from build123d import *

# Parameters (mm, degrees)
SKETCH2_W              = 127
SKETCH2_H              = 127
BOSS_EXTRUDE1_DEPTH    = 12.7
SKETCH3_W              = 38.1
SKETCH3_H              = 4.04158002
CUT_EXTRUDE2_DEPTH     = 128
F_10_0MM_DOWEL_HOLE1_D = 8.382
CUT_EXTRUDE4_DEPTH     = 13.7


with BuildPart() as part:
    # Sketch2 → Boss-Extrude1 (new body)
    with BuildSketch(Plane(origin=(0, 0, 0), x_dir=(1, 0, 0), z_dir=(0, 1, 0))):
        Rectangle(SKETCH2_W, SKETCH2_H)
    extrude(amount=BOSS_EXTRUDE1_DEPTH)

    # Sketch3 → Cut-Extrude2 (cut, through all)
    with BuildSketch(Plane.XY.offset(63.5)):
        with Locations((-44.45, 10.67920999)):
            Rectangle(SKETCH3_W, SKETCH3_H)
        with Locations((44.45, 10.67920999)):
            Rectangle(SKETCH3_W, SKETCH3_H)
    extrude(amount=-CUT_EXTRUDE2_DEPTH, mode=Mode.SUBTRACT)

    # Ø10.0mm Dowel Hole1 (through all)
    with Locations(Plane(origin=(0, 0, 0), x_dir=(-1, 0, 0), z_dir=(0, -1, 0))):
        with Locations((-44.45, 43.18), (-44.45, -4.572), (-44.45, -42.672), (44.45, 43.18), (44.45, -4.572), (44.45, -42.672)):
            Hole(F_10_0MM_DOWEL_HOLE1_D / 2)

    # Sketch10 → Cut-Extrude4 (cut, through all)
    with BuildSketch(Plane(origin=(0, 0, 0), x_dir=(-1, 0, 0), z_dir=(0, -1, 0))):
        with BuildLine():
            Line((7.62, -11.938), (7.62, -36.322))
            ThreePointArc((7.62, -36.322), (0, -43.942), (-7.62, -36.322))
            Line((-7.62, -36.322), (-7.62, -11.938))
            ThreePointArc((-7.62, -11.938), (0, -4.318), (7.62, -11.938))
        make_face()
    extrude(amount=-CUT_EXTRUDE4_DEPTH, mode=Mode.SUBTRACT)


solid = part.part
Can you work these out from the model? Positions are in its coordinate system, mm. A direction names the side the tool comes from. Round coordinates to 2 decimals unless told otherwise and drop trailing zeros. Write each loop counter-clockwise with the first axis right and the second up, starting at its lowest first coordinate (ties: lowest second). Pieces come first, ordered by that corner, then holes. Notation, with made-up numbers: (-10.5, -37.5) -> (41.5, -37.5) arc R30 ccw to (41.5, -7.5) -> close; hole circle Ø10 at (80.5, 63.25). An arc over 180 degrees is marked (long way). One line per question, with ' | ' between items. Start each with the question number.
1) If we mould it in two halves opening along Z, with no side actions, what happens to faces 1 (the flat face through (-1, 5, -63.5)), 2 (the flat face through (63.5, 4, 1)), 3 (the cylindrical face through (-47.78, 4.39, 45.22))? For each: released by +Z, released by -Z, zero draft, split by the parting line, or undercut.
2) Suppose I cut it at B-B on x = 0. Write out the boundary of the cut face in (y, z), then the cut area to 3 significant figures.
3) On a 3-axis mill with a long thin cutter (end or side, diameter ignored), from which of +Z, -Z, +X, -X, +Y, -Y can I reach the whole of each face in a straight line? I mean faces 4 (the flat face through (40, 8.658, 1)), 5 (the flat face through (0, 12.7, -1)), 6 (the cylindrical face through (0.17, 6.26, 4.32)), 7 (the flat face through (-49, 8.658, 1)), 8 (the flat face through (-1, 0, -1)). Say none if no direction works.
4) I'm going to push flat-ended pins straight in: P1, Ø2, axis at y = 11, z = -21.5, coming from the -X side; P2, Ø7.5, axis at x = -44.45, z = 42.672, coming from the -Y side; P3, Ø12, axis at x = 5, z = 9.5, coming from the -Y side; P4, Ø13.5, axis at x = -44.45, z = 4.572, coming from the +Y side. Where does each tip first touch, or does it pass through?
5) Suppose I cut it at D-D on x = -44.45. Write out the boundary of the cut face in (y, z).
6) Suppose I cut it at C-C on y = 11. Write out the boundary of the cut face in (x, z), then the cut area to 3 significant figures.
7) I need wall thicknesses on line 1 (Z direction, x = -44.45, y = 3); line 2 (X direction, y = 8.25, z = 12); line 3 (X direction, y = 12.25, z = 26). Which ranges of each line are inside material? Lowest first, please. Write a range as [from, to].
8) Suppose I cut it at A-A on z = 20.5. Write out the boundary of the cut face in (x, y).
Return value:
1) face 1: released by -Z | face 2: zero draft | face 3: undercut
2) outline: (0, -63.5) -> (12.7, -63.5) -> (12.7, 4.32) -> (0, 4.32) -> close; (0, 43.94) -> (12.7, 43.94) -> (12.7, 63.5) -> (0, 63.5) -> close | area: 1,110 mm2
3) face 4: +Z, -Z, +X, +Y | face 5: +Z, -Z, +X, -X, +Y | face 6: +Y, -Y | face 7: +Z, -Z, -X, +Y | face 8: +Z, -Z, +X, -X, -Y
4) P1: stops at x = -25.4 | P2: passes through | P3: stops at y = 0 | P4: stops at y = 8.66
5) outline: (0, -63.5) -> (8.66, -63.5) -> (8.66, -47.37) -> (0, -47.37) -> close; (0, -38.99) -> (8.66, -38.99) -> (8.66, 0.38) -> (0, 0.38) -> close; (0, 8.76) -> (8.66, 8.76) -> (8.66, 38.48) -> (0, 38.48) -> close; (0, 46.86) -> (8.66, 46.86) -> (8.66, 63.5) -> (0, 63.5) -> close
6) outline: (-25.4, -63.5) -> (25.4, -63.5) -> (25.4, 63.5) -> (-25.4, 63.5) -> close; hole (-7.62, 11.94) arc R7.62 ccw to (7.62, 11.94) -> (7.62, 36.32) arc R7.62 ccw to (-7.62, 36.32) -> close | area: 5,900 mm2
7) line 1: z = [-63.5, -47.37], [-38.99, 0.38], [8.76, 38.48], [46.86, 63.5] | line 2: x = [-63.5, -7.62], [7.62, 63.5] | line 3: x = [-25.4, -7.62], [7.62, 25.4]
8) outline: (-63.5, 0) -> (-7.62, 0) -> (-7.62, 12.7) -> (-25.4, 12.7) -> (-25.4, 8.66) -> (-63.5, 8.66) -> close; (7.62, 0) -> (63.5, 0) -> (63.5, 8.66) -> (25.4, 8.66) -> (25.4, 12.7) -> (7.62, 12.7) -> close
